```python
from build123d import *

# Parameters (mm, degrees)
SKETCH1_R           = 1.5
SKETCH1_R_2         = 1.75
BOSS_EXTRUDE1_DEPTH = 2


with BuildPart() as part:
    # Sketch1 → Boss-Extrude1 (new body)
    with BuildSketch(Plane.XY):
        with BuildLine():
            Line((-122.6, 12), (122.6, 12))
            ThreePointArc((122.6, 12), (134.6, 0), (122.6, -12))
            Line((122.6, -12), (-122.6, -12))
            ThreePointArc((-122.6, -12), (-134.6, 0), (-122.6, 12))
        make_face()
        with Locations((-122.6, 0)):
            Circle(SKETCH1_R, mode=Mode.SUBTRACT)
        Circle(SKETCH1_R_2, mode=Mode.SUBTRACT)
        with Locations((122.6, 0)):
            Circle(SKETCH1_R, mode=Mode.SUBTRACT)
    extrude(amount=BOSS_EXTRUDE1_DEPTH)


solid = part.part
```
The listing builds one solid part. Answer for the finished solid, in the listing's coordinates (mm). Give positions to 0.01 mm unless a question says otherwise; leave off trailing zeros. Order: outer loops, then holes, each group sorted by start corner. A loop starts at its lowest first (then second) coordinate and runs counter-clockwise, first axis right, second up. Notation, with made-up numbers: M 77,27 L 89,27 A20 ccw 89,40 Z; hole C 52,53 d7. An arc over 180 degrees is marked long. Put each result on its own line as item: value. Start each with the question number.
Item 1: The part is cut by section B-B, the plane y = 8.25. Determine the outline of the cut face in (x, z).
Item 2: The part is cut by section A-A, the plane z = 1.1. Determine the outline of the cut face in (x, y).
Item 3: The part is cut by section C-C, the plane y = -6.75. Determine the outline of the cut face in (x, z), and give its area (3 significant figures).
Item 4: Find the intervals of material crossed by line 1 along Y through (x, z) = (-122.6, 1); line 2 along Y through (x, z) = (0, 0.6); line 3 along X through (y, z) = (-8, 0.85), in increasing order.
Answer key:
1. outline: M -131.31,0 L 131.31,0 L 131.31,2 L -131.31,2 Z
2. outline: M -122.6,-12 L 122.6,-12 A12 ccw 122.6,12 L -122.6,12 A12 ccw Z; hole C -122.6,0 d3; hole C 0,0 d3.5; hole C 122.6,0 d3
3. outline: M -132.52,0 L 132.52,0 L 132.52,2 L -132.52,2 Z
3. area: 530 mm²
4. line 1: y = -12 to -1.5, 1.5 to 12
4. line 2: y = -12 to -1.75, 1.75 to 12
4. line 3: x = -131.54 to 131.54
